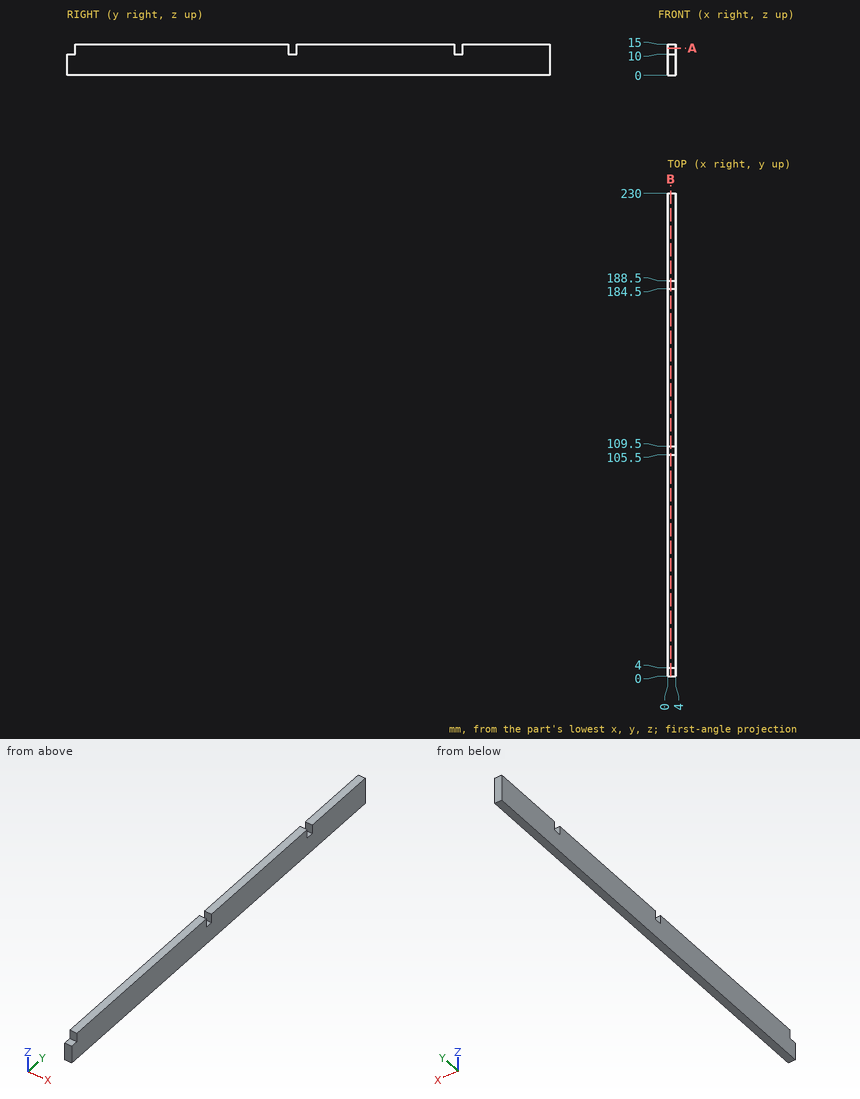
Input: dimensioned drawing with shaded views. Units: mm. Origin: part minimum x, y, z. Round coordinates to 2 decimals unless told otherwise and drop trailing zeros. Loops run counter-clockwise (first coordinate to the right, second up) from the corner with the lowest first, then second, coordinate; pieces in that order, holes last. Notation, with made-up numbers: (22.5, 10.5) -> (31.5, 10.5) arc R11 ccw to (31.5, 14.5) -> close; hole circle Ø5 at (-9.75, 60.25). An arc over 180 degrees is marked (long way). Use one line per item in the form item = value. Start each with the question number.
1) Section B-B on x = 1.4. Output: boundary loops of the cut face in (y, z), then the cut area to 3 significant figures.
2) First-contact query: P1, Ø2, axis at x = 2, y = 107, coming from the +Z side; P2, Ø2, axis at x = 1.5, z = 12, coming from the -Y side. Flat tips, straight axial feed; report the tip coordinate or a pass-through.
3) Section A-A on z = 13. Output: boundary loops of the cut face in (x, y).
4) Line query: L1, parallel to Y at x = 2.1, z = 12. Output: solid intervals per line, ascending.
Response:
q1.outline = (0, 0) -> (230, 0) -> (230, 15) -> (188.5, 15) -> (188.5, 10) -> (184.5, 10) -> (184.5, 15) -> (109.5, 15) -> (109.5, 10) -> (105.5, 10) -> (105.5, 15) -> (4, 15) -> (4, 10) -> (0, 10) -> close
q1.area = 3,390 mm^2
q2.P1 = 10
q2.P2 = 4
q3.outline = (0, 4) -> (4, 4) -> (4, 105.5) -> (0, 105.5) -> close; (0, 109.5) -> (4, 109.5) -> (4, 184.5) -> (0, 184.5) -> close; (0, 188.5) -> (4, 188.5) -> (4, 230) -> (0, 230) -> close
q4.L1 = 4 to 105.5, 109.5 to 184.5, 188.5 to 230
